from build123d import *

# Parameters (mm, degrees)
SKETCH1_W                    = 62
SKETCH1_H                    = 19
SKETCH1_R                    = 2.25
BASE_FLANGE1_DEPTH           = 1.5
EDGE_FLANGE1_STRIP_W         = 7.4732
EDGE_FLANGE1_STRIP_H         = 1.5
EDGE_FLANGE1_STRIP_CUT_DEPTH = 19
EDGE_FLANGE1_DEPTH           = 19
EDGE_FLANGE2_STRIP_W         = 7.4732
EDGE_FLANGE2_STRIP_H         = 1.5
EDGE_FLANGE2_STRIP_CUT_DEPTH = 19
EDGE_FLANGE2_DEPTH           = 19
SKETCH12_R                   = 2.5
CUT_EXTRUDE1_DEPTH           = 69.317274536


# Sheet-metal steps are written as plain solids
with BuildPart() as part:
    # Sketch1 → Base-Flange1 (new body)
    with BuildSketch(Plane(origin=(0, 0, 0), x_dir=(1, 0, 0), z_dir=(0, 1, 0))):
        with Locations((31, 9.5)):
            Rectangle(SKETCH1_W, SKETCH1_H)
        with Locations(Location((15, 9.5, 0), (0, 0, 270))):
            Circle(SKETCH1_R, mode=Mode.SUBTRACT)
        with Locations(Location((47, 9.5, 0), (0, 0, 270))):
            Circle(SKETCH1_R, mode=Mode.SUBTRACT)
    extrude(amount=-BASE_FLANGE1_DEPTH)

    # Edge-Flange1 strip (across the edge) → Edge-Flange1 strip cut (cut)
    with BuildSketch(Plane.XY.offset(-19)):
        with Locations((-1.5, -0.75)):
            Rectangle(EDGE_FLANGE1_STRIP_W, EDGE_FLANGE1_STRIP_H)
    extrude(amount=EDGE_FLANGE1_STRIP_CUT_DEPTH, mode=Mode.SUBTRACT)

    # Edge-Flange1 section (across the edge) → Edge-Flange1 (add)
    with BuildSketch(Plane.XY.offset(-19)):
        with BuildLine():
            Line((0, 0.7366), (0, 21.5))
            Line((0, 21.5), (1.5, 21.5))
            Line((1.5, 21.5), (1.5, 0.7366))
            ThreePointArc((1.5, 0.7366), (1.715745145, 0.215745145), (2.2366, 0))
            Line((2.2366, 0), (2.2366, -1.5))
            ThreePointArc((2.2366, -1.5), (0.655084973, -0.844915027), (0, 0.7366))
        make_face()
    extrude(amount=EDGE_FLANGE1_DEPTH)

    # Edge-Flange2 strip (across the edge) → Edge-Flange2 strip cut (cut)
    with BuildSketch(Plane(origin=(62, 0, 0), x_dir=(-1, 0, 0), z_dir=(0, 0, -1))):
        with Locations((-1.5, -0.75)):
            Rectangle(EDGE_FLANGE2_STRIP_W, EDGE_FLANGE2_STRIP_H)
    extrude(amount=EDGE_FLANGE2_STRIP_CUT_DEPTH, mode=Mode.SUBTRACT)

    # Edge-Flange2 section (across the edge) → Edge-Flange2 (add)
    with BuildSketch(Plane(origin=(62, 0, 0), x_dir=(-1, 0, 0), z_dir=(0, 0, -1))):
        with BuildLine():
            Line((0, 0.7366), (0, 21.5))
            Line((0, 21.5), (1.5, 21.5))
            Line((1.5, 21.5), (1.5, 0.7366))
            ThreePointArc((1.5, 0.7366), (1.715745145, 0.215745145), (2.2366, 0))
            Line((2.2366, 0), (2.2366, -1.5))
            ThreePointArc((2.2366, -1.5), (0.655084973, -0.844915027), (0, 0.7366))
        make_face()
    extrude(amount=EDGE_FLANGE2_DEPTH)

    # Sketch12 → Cut-Extrude1 (cut, through all)
    with BuildSketch(Plane(origin=(62, 0, 0), x_dir=(0, 0, -1), z_dir=(1, 0, 0))):
        with Locations(Location((9.5, 14.5, 0), (0, 0, 90))):
            Circle(SKETCH12_R)
        with BuildLine():
            Line((0, 11.7366), (-3.023600292, 11.7366))
            Line((-3.023600292, 11.7366), (-3.023600292, 23.521513474))
            Line((-3.023600292, 23.521513474), (21.663618521, 23.521513474))
            Line((21.663618521, 23.521513474), (21.663618521, 11.7366))
            Line((21.663618521, 11.7366), (19, 11.7366))
            ThreePointArc((19, 11.7366), (9.5, 21.2366), (0, 11.7366))
        make_face()
    extrude(amount=-CUT_EXTRUDE1_DEPTH, mode=Mode.SUBTRACT)


solid = part.part
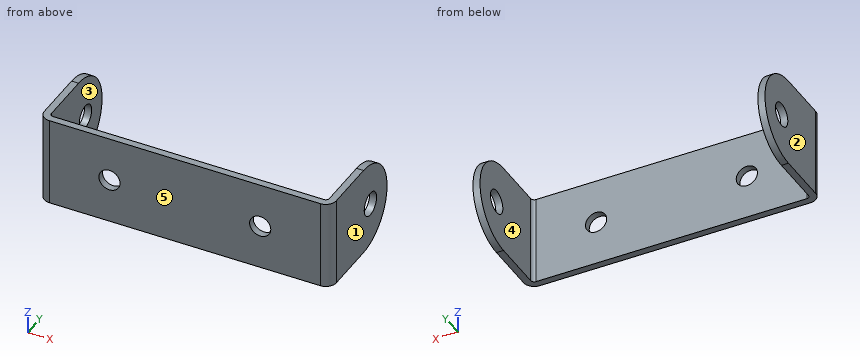
Could you check a few things on this model? Use its own coordinates, in mm. Face numbers are marked on the shaded views. A direction names the side the tool comes from. Give positions to 0.01 mm unless a question says otherwise; leave off trailing zeros. Write each loop counter-clockwise with the first axis right and the second up, starting at its lowest first coordinate (ties: lowest second). Pieces come first, ordered by that corner, then holes. Notation, with made-up numbers: (30.25, -8.75) -> (65.25, -8.75) arc R19 cw to (65.25, 22.25) -> close; hole circle Ø8 at (50, -17). An arc over 180 degrees is marked (long way). Answer as CSV lines item,"result". Start each with the question number.
(1) I'm going to push flat-ended pins straight in: pin 1 Ø10 at (x, y) = (9.5, 10) entering from +Z; pin 2 Ø3 at (x, z) = (26, -4.5) entering from +Y. Where does each tip first touch, or does it pass through?
(2) If we section it at A-A, the plane x = 15: Write out the boundary of the cut face in (y, z).
(3) If we section it at B-B, the plane z = -9.5: Write out the boundary of the cut face in (x, y), and give its area (3 significant figures).
(4) Which directions (+Z, -Z, +X, -X, +Y, -Y) give clear straight access to the entire face, cutting with the end or side of a thin tool? Please do the marked faces 4 and 5.
(5) If we section it at D-D, the plane z = -5.75: Write out the boundary of the cut face in (x, y), and give its area (3 significant figures).
(6) Please list where these lines run through material, in increasing order: line 1 (X direction, y = 1.75, z = -2); line 2 (X direction, y = -0.45, z = -9.5); line 3 (Y direction, x = 22, z = -16.5).
(7) If we section it at C-C, the plane y = 14.5: Write out the boundary of the cut face in (x, z), and give its area (3 significant figures).
(8) If we mould it in two halves opening along X, with no side actions, what happens to the marked faces 1, 2 and 3? For each: +X half, -X half, draft (parallel to the pull), parting line (faces both ways), or undercut.
Answer list:
1,pin 1,"through"
1,pin 2,"y = 0"
2,outline,"(-1.5, -19) -> (0, -19) -> (0, -11.75) -> (-1.5, -11.75) -> close; (-1.5, -7.25) -> (0, -7.25) -> (0, 0) -> (-1.5, 0) -> close"
3,outline,"(0, 0.74) arc R2.24 ccw to (2.24, -1.5) -> (12.75, -1.5) -> (12.75, 0) -> (2.24, 0) arc R0.74 cw to (1.5, 0.74) -> (1.5, 12) -> (0, 12) -> close; (0, 17) -> (1.5, 17) -> (1.5, 21.24) -> (0, 21.24) -> close; (17.25, -1.5) -> (44.75, -1.5) -> (44.75, 0) -> (17.25, 0) -> close; (49.25, -1.5) -> (59.76, -1.5) arc R2.24 ccw to (62, 0.74) -> (62, 12) -> (60.5, 12) -> (60.5, 0.74) arc R0.74 cw to (59.76, 0) -> (49.25, 0) -> close; (60.5, 17) -> (62, 17) -> (62, 21.24) -> (60.5, 21.24) -> close"
3,area,"126 mm^2"
4,face 4,"+Z, -Z, +Y"
4,face 5,"+Z, -Z, +X, -X, -Y"
5,outline,"(0, 0.74) arc R2.24 ccw to (2.24, -1.5) -> (59.76, -1.5) arc R2.24 ccw to (62, 0.74) -> (62, 20.47) -> (60.5, 20.47) -> (60.5, 0.74) arc R0.74 cw to (59.76, 0) -> (2.24, 0) arc R0.74 cw to (1.5, 0.74) -> (1.5, 20.47) -> (0, 20.47) -> close"
5,area,"152 mm^2"
6,line 1,"0 to 1.5, 60.5 to 62"
6,line 2,"0.34 to 12.75, 17.25 to 44.75, 49.25 to 61.66"
6,line 3,"-1.5 to 0"
7,outline,"(0, -18.59) -> (1.5, -18.59) -> (1.5, -12) -> (0, -12) -> close; (0, -7) -> (1.5, -7) -> (1.5, -0.41) -> (0, -0.41) -> close; (60.5, -18.59) -> (62, -18.59) -> (62, -12) -> (60.5, -12) -> close; (60.5, -7) -> (62, -7) -> (62, -0.41) -> (60.5, -0.41) -> close"
7,area,"39.5 mm^2"
8,face 1,"+X half"
8,face 2,"-X half"
8,face 3,"undercut"
